```python
from build123d import *

# Parameters (mm, degrees)
SKETCH1_R               = 20
BOSS_EXTRUDE1_DEPTH     = 52.8796
SKETCH2_R               = 20
SKETCH2_R_2             = 18
CUT_EXTRUDE2_DEPTH      = 1.85
SKETCH6_R               = 20
BOSS_EXTRUDE2_DEPTH     = 5
SKETCH7_R               = 15
CUT_EXTRUDE3_DEPTH      = 1
CUT_EXTRUDE3_DEPTH_BACK = 116.7592


with BuildPart() as part:
    # Sketch1 → Boss-Extrude1 (new body)
    with BuildSketch(Plane.XY):
        Circle(SKETCH1_R)
    extrude(amount=BOSS_EXTRUDE1_DEPTH)

    # Sketch2 → Cut-Extrude2 (cut)
    with BuildSketch(Plane.XY.offset(52.8796)):
        Circle(SKETCH2_R)
        Circle(SKETCH2_R_2, mode=Mode.SUBTRACT)
    extrude(amount=-CUT_EXTRUDE2_DEPTH, mode=Mode.SUBTRACT)

    # Sketch6 → Boss-Extrude2 (add)
    with BuildSketch(Plane.XY.offset(52.8796)):
        Circle(SKETCH6_R)
    extrude(amount=BOSS_EXTRUDE2_DEPTH)

    # Mirror2: part across plane


with BuildPart() as part_1:
    add(part.part)
    add(part.part.mirror(Plane.XY))

    # Sketch7 → Cut-Extrude3 (cut, two sides)
    with BuildSketch(Plane(origin=(0, 0, -57.8796), x_dir=(-1, 0, 0), z_dir=(0, 0, -1))) as cut_extrude3_sk:
        Circle(SKETCH7_R)
    extrude(amount=CUT_EXTRUDE3_DEPTH, mode=Mode.SUBTRACT)
    extrude(cut_extrude3_sk.sketch, amount=-CUT_EXTRUDE3_DEPTH_BACK, mode=Mode.SUBTRACT)


solid = part_1.part
```
Here's how the part is built. I have some questions about the finished solid (model axes, mm). A direction names the side the tool comes from. Coordinates: 2 decimals unless noted, no trailing zeros. Order: outer loops, then holes, each group sorted by start corner. A loop starts at its lowest first (then second) coordinate and runs counter-clockwise, first axis right, second up.
Item 1: If we section it at A-A, the plane y = 0: List the corners of the cut face in (x, z) for me.
Response values:
outline: (-20, -57.88) - (-15, -57.88) - (-15, 57.88) - (-20, 57.88) - (-20, 52.88) - (-18, 52.88) - (-18, 51.03) - (-20, 51.03) - (-20, -51.03) - (-18, -51.03) - (-18, -52.88) - (-20, -52.88) - close; (15, -57.88) - (20, -57.88) - (20, -52.88) - (18, -52.88) - (18, -51.03) - (20, -51.03) - (20, 51.03) - (18, 51.03) - (18, 52.88) - (20, 52.88) - (20, 57.88) - (15, 57.88) - close
Item 2: If we section it at C-C, the plane z = 3.5: List the corners of the cut face in (x, y) for me.
Response values:
outline: circle Ø40 at (0, 0); hole circle Ø30 at (0, 0)
Item 3: I need wall thicknesses on probe 1 along Y at (x, z) = (0, -28); probe 2 along X at (y, z) = (4, 48); probe 3 along X at (y, z) = (9, -3). Which ranges of each line are inside material? Lowest first, please.
Response values:
probe 1: y = -20 to -15, 15 to 20
probe 2: x = -19.6 to -14.46, 14.46 to 19.6
probe 3: x = -17.86 to -12, 12 to 17.86
Item 4: I'm going to push flat-ended pins straight in: pin 1 Ø6 at (x, z) = (11.5, 27.5) entering from -Y; pin 2 Ø1.5 at (x, z) = (-1, 18) entering from -Y; pin 3 Ø12 at (y, z) = (-7.5, 14) entering from +X; pin 4 Ø20 at (x, y) = (8.5, 6.5) entering from +Z. Where does each tip first touch, or does it pass through?
Response values:
pin 1: stops at y = -18.1
pin 2: stops at y = -20
pin 3: stops at x = 19.94
pin 4: stops at z = 57.88
Item 5: Thinking about a two-plate mould opening in Z: for faces 3 (the face through (14.985, 0.66, -0.81)), 4 (the face through (3, 15, -57.88)), 5 (the face through (-2.343, 17.847, 51.968)), 6 (the face through (-18, 3, -51.03)), which applies, pulls with the +Z half, pulls with the -Z half, needs draft (parallel to the pull), parting line crosses it, or undercut?
Response values:
face 3: needs draft
face 4: pulls with the -Z half
face 5: undercut
face 6: undercut
Item 6: Which directions (+Z, -Z, +X, -X, +Y, -Y) give clear straight access to the entire face, cutting with the end or side of a thin tool? Please do faces 1 (the face through (-18, 3, -52.88)), 2 (the face through (-4.336, -19.524, -55.345)).
Response values:
face 1: none
face 2: +Z, -Z
